Study the drawing (mm; zero at the part's minimum x, y, z) and answer. Coordinates: 2 decimals unless noted, no trailing zeros. Order: outer loops, then holes, each group sorted by start corner. A loop starts at its lowest first (then second) coordinate and runs counter-clockwise, first axis right, second up. Notation, with made-up numbers: (-8, 5) -> (39, 5) arc R15 cw to (39, 10) -> close; hole circle Ø5 at (1, 36.25). An arc over 180 degrees is marked (long way). One line per question, with ' | ' between items.
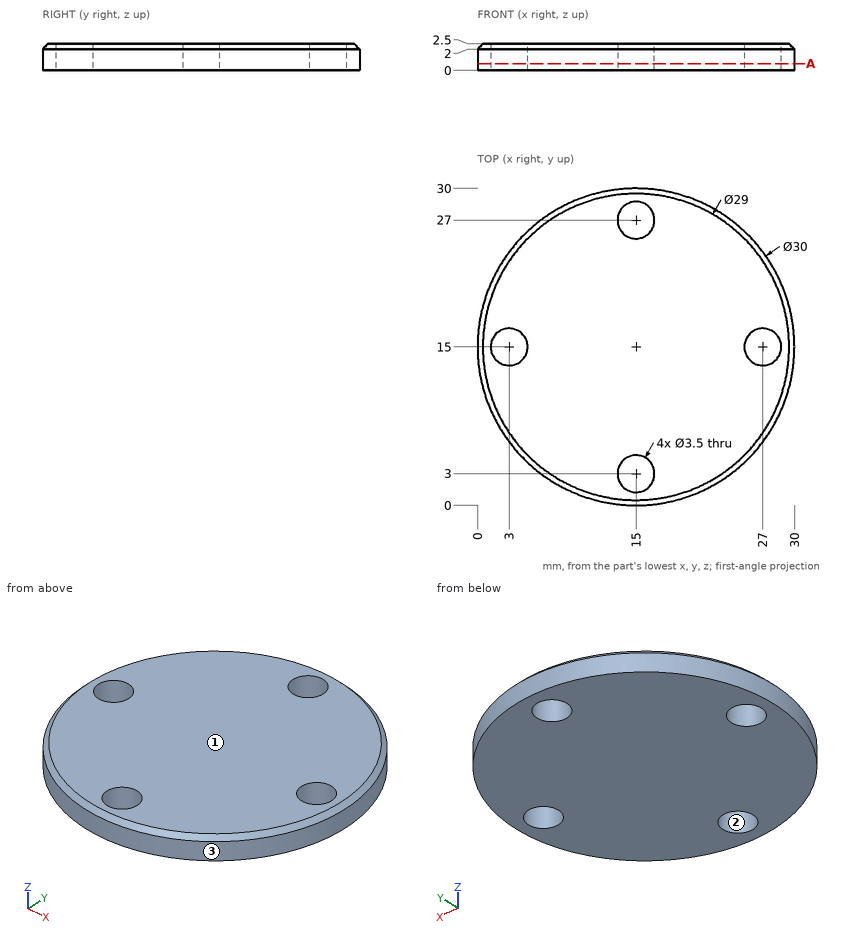
Item 1: Determine the mould class of the marked faces 1, 2 and 3 for opening direction X: pulls with the +X half, pulls with the -X half, needs draft (parallel to the pull), parting line crosses it, or undercut.
Computed values:
face 1: needs draft | face 2: undercut | face 3: parting line crosses it
Item 2: Each of these flat-tipped pins is pushed along its axis until it touches: pin 1 Ø5.5 at (x, y) = (27, 15) entering from +Z; pin 2 Ø1 at (x, z) = (23, 1) entering from -Y; pin 3 Ø1 at (y, z) = (26, 0.5) entering from -X. Where does it stop, or does it pass through?
Computed values:
pin 1: stops at z = 2.5 | pin 2: stops at y = 2.01 | pin 3: stops at x = 4.29
Item 3: Find the intervals of material crossed by L1, parallel to Y at x = 15, z = 0.75; L2, parallel to Y at x = 2.5, z = 2.3; L3, parallel to Y at x = 3, z = 1.3, in increasing order.
Computed values:
L1: y = 0 to 1.25, 4.75 to 25.25, 28.75 to 30 | L2: y = 7.26 to 13.32, 16.68 to 22.74 | L3: y = 6 to 13.25, 16.75 to 24
Item 4: Section A-A, the plane z = 0.65 is taken. Give the vertices of the cut face in (x, y).
Computed values:
outline: circle Ø30 at (15, 15); hole circle Ø3.5 at (3, 15); hole circle Ø3.5 at (15, 3); hole circle Ø3.5 at (15, 27); hole circle Ø3.5 at (27, 15)
